```python
from build123d import *

# Parameters (mm, degrees)
SKETCH1_W                               = 325
SKETCH1_H                               = 260
BOSS_EXTRUDE1_DEPTH                     = 39
CBORE_FOR_M5_HEX_HEAD_BOLT1_D           = 5.5
CBORE_FOR_M5_HEX_HEAD_BOLT1_DEPTH       = 30
CBORE_FOR_M5_HEX_HEAD_BOLT1_CBORE_D     = 12.238
CBORE_FOR_M5_HEX_HEAD_BOLT1_CBORE_DEPTH = 3.5
CBORE_FOR_M5_HEX_HEAD_BOLT1_TIP         = 1.652366702
SKETCH10_W                              = 39
SKETCH10_H                              = 260
CUT_EXTRUDE2_DEPTH                      = 25
SKETCH11_W                              = 25
SKETCH11_H                              = 247
CUT_EXTRUDE3_DEPTH                      = 14
F_6_0MM_DOWEL_HOLE1_D                   = 6
F_6_0MM_DOWEL_HOLE1_DEPTH               = 15
F_6_0MM_DOWEL_HOLE1_TIP                 = 1.802581857
CUT_EXTRUDE4_DEPTH                      = 222.463315247
CUT_EXTRUDE4_DEPTH_BACK                 = 222.463315247
SKETCH15_W                              = 25
SKETCH15_H                              = 14


with BuildPart() as part:
    # Sketch1 → Boss-Extrude1 (new body)
    with BuildSketch(Plane(origin=(0, 0, 0), x_dir=(0, 0, -1), z_dir=(1, 0, 0))):
        with Locations((-12.5, 0)):
            Rectangle(SKETCH1_W, SKETCH1_H)
    extrude(amount=BOSS_EXTRUDE1_DEPTH)

    # CBORE for M5 Hex Head Bolt1
    with Locations(Plane(origin=(39, 0, 0), x_dir=(0, 0, -1), z_dir=(1, 0, 0))):
        with Locations((133, -101), (133, 76), (-158, 76), (-158, -101)):
            CounterBoreHole(CBORE_FOR_M5_HEX_HEAD_BOLT1_D / 2, CBORE_FOR_M5_HEX_HEAD_BOLT1_CBORE_D / 2, CBORE_FOR_M5_HEX_HEAD_BOLT1_CBORE_DEPTH, depth=CBORE_FOR_M5_HEX_HEAD_BOLT1_DEPTH)
            with Locations((0, 0, -(CBORE_FOR_M5_HEX_HEAD_BOLT1_DEPTH + CBORE_FOR_M5_HEX_HEAD_BOLT1_TIP / 2))):  # 118° drill point
                Cone(0, CBORE_FOR_M5_HEX_HEAD_BOLT1_D / 2, CBORE_FOR_M5_HEX_HEAD_BOLT1_TIP, mode=Mode.SUBTRACT)

    # Sketch10 → Cut-Extrude2 (cut)
    with BuildSketch(Plane(origin=(0, 0, 0), x_dir=(0, 0, -1), z_dir=(1, 0, 0))):
        with Locations((130.5, 0)):
            Rectangle(SKETCH10_W, SKETCH10_H)
        with Locations((-155.5, 0)):
            Rectangle(SKETCH10_W, SKETCH10_H)
    extrude(amount=CUT_EXTRUDE2_DEPTH, mode=Mode.SUBTRACT)

    # Sketch11 → Cut-Extrude3 (cut)
    with BuildSketch(Plane(origin=(0, 130, 0), x_dir=(1, 0, 0), z_dir=(0, 1, 0))):
        with Locations((12.5, -12.5)):
            Rectangle(SKETCH11_W, SKETCH11_H)
    extrude(amount=-CUT_EXTRUDE3_DEPTH, mode=Mode.SUBTRACT)

    # Ø6.0mm Dowel Hole1
    with Locations(Plane(origin=(0, 116, 0), x_dir=(1, 0, 0), z_dir=(0, 1, 0))):
        with Locations((14, 71.5), (14, -96.5)):
            Hole(F_6_0MM_DOWEL_HOLE1_D / 2, depth=F_6_0MM_DOWEL_HOLE1_DEPTH)
            with Locations((0, 0, -(F_6_0MM_DOWEL_HOLE1_DEPTH + F_6_0MM_DOWEL_HOLE1_TIP / 2))):  # 118° drill point
                Cone(0, F_6_0MM_DOWEL_HOLE1_D / 2, F_6_0MM_DOWEL_HOLE1_TIP, mode=Mode.SUBTRACT)

    # Sketch15 → Cut-Extrude4 (cut, two sides: drawn at the far end of the back side and taken through both)
    with BuildSketch(Plane.XY.offset(-CUT_EXTRUDE4_DEPTH_BACK)):
        with Locations((12.5, -123)):
            Rectangle(SKETCH15_W, SKETCH15_H)
    extrude(amount=CUT_EXTRUDE4_DEPTH + CUT_EXTRUDE4_DEPTH_BACK, mode=Mode.SUBTRACT)


solid = part.part
```
The listing builds one solid part. Answer for the finished solid, in the listing's coordinates (mm). A direction names the side the tool comes from. Coordinates: 2 decimals unless noted, no trailing zeros. Loops run counter-clockwise (first coordinate to the right, second up) from the corner with the lowest first, then second, coordinate; pieces in that order, holes last. Notation, with made-up numbers: M 39.5,8.5 L 52.5,8.5 A27 ccw 52.5,43.5 Z; hole C 30.5,80 d11. An arc over 180 degrees is marked long. Answer as a JSON object with one key per item and string values. Group by question number.
Item 1: Each of these flat-tipped pins is pushed along its axis until it touches: P1, Ø19.5, axis at y = -101, z = 158, coming from the -X side; P2, Ø1, axis at y = 96, z = -102.5, coming from the -X side; P3, Ø7, axis at y = -101, z = 158, coming from the +X side; P4, Ø3.5, axis at y = 76, z = 158, coming from the -X side. Where does it stop, or does it pass through?
Item 2: Section B-B (z = 107) is taken. Write down the section's boundary in (x, y).
Item 3: Which of the six approach directions +Z, -Z, +X, -X, +Y, -Y give full straight-line access (tool end or side, diameter ignored) to faces 1 (the face through (37.274, 80.136, -128.49)), 2 (the face through (12, -116, 11)), 3 (the face through (12, -2, -111)), 4 (the face through (12, -2, 136))?
Item 4: Section A-A (y = -82.5) is taken. Write down the section's boundary in (x, z), and give its area (3 significant figures).
Item 5: Determine the mould class of faces 5 (the face through (35.5, 75, 155)), 6 (the face through (32, -2, -150)), 7 (the face through (35.5, 73, -134)), 8 (the face through (12, 116, 11)) for opening direction Z: +Z half, -Z half, draft (parallel to the pull), parting line (faces both ways), or undercut.
Item 6: Section C-C (x = 4) is taken. Write down the section's boundary in (y, z), and give its area (3 significant figures).
Item 7: Consider L1, parallel to Y at x = 36.35, z = 158; L2, parallel to Y at x = 29, z = 158; L3, parallel to Z at x = 14, y = 106. Determine where each line is inside the solid, lowest interval first.
Solved:
{
 "1": {"P1": "stops at x = 25", "P2": "stops at x = 0", "P3": "stops at x = 35.5", "P4": "passes through"},
 "2": {"outline": "M 0,-116 L 25,-116 L 25,-130 L 39,-130 L 39,130 L 25,130 L 25,116 L 0,116 Z"},
 "3": {"face 1": "+X", "face 2": "+Z, -Z, -X, -Y", "face 3": "-Z, -X, +Y, -Y", "face 4": "+Z, -X, +Y, -Y"},
 "4": {"outline": "M 0,-111 L 25,-111 L 25,-150 L 39,-150 L 39,175 L 25,175 L 25,136 L 0,136 Z", "area": "10,700 mm2"},
 "5": {"face 5": "undercut", "face 6": "-Z half", "face 7": "undercut", "face 8": "draft"},
 "6": {"outline": "M -116,-111 L 116,-111 L 116,136 L -116,136 Z", "area": "57,300 mm2"},
 "7": {"L1": "y = -130 to -107.12, -94.88 to 69.88, 82.12 to 130", "L2": "y = -130 to -103.75, -98.25 to 73.25, 78.75 to 130", "L3": "z = -111 to -74.5, -68.5 to 93.5, 99.5 to 136"}
}
